Input: part model. Units: mm. Frame: model coordinates. Round coordinates to 2 decimals unless told otherwise and drop trailing zeros. Loops run counter-clockwise (first coordinate to the right, second up) from the corner with the lowest first, then second, coordinate; pieces in that order, holes last. Notation, with made-up numbers: (71, 9) - (98, 9) arc R10 ccw to (98, 13) - close; hole circle Ø10 at (-21.75, 8). An arc over 180 degrees is marked (long way). One line per question, with ' | ' between items. Start each with the question number.
Item 1: Material intervals for line 1 along Y through (x, z) = (0, -23.5); line 2 along Z through (x, y) = (-54.5, -18); line 3 along X through (y, z) = (11, -49.5), sorted ascending.
Item 2: First-contact query: pin 1 (6 mm diameter, centred on y = 30, z = -12.5, fed in from +X); pin 2 (3 mm diameter, centred on y = -22.5, z = -55, fed in from -X); pin 3 (1.5 mm diameter, centred on x = -29, y = -27, fed in from -Z). Flat tips, straight axial feed; report the tip coordinate or a pass-through.
Item 3: Section C-C, the plane z = 4. Return loops of the section in (x, y) (1 decimal), plus the area to 3 significant figures.
Item 4: Section A-A, the plane y = 0. Return loops of the section in (x, z), plus the area to 3 significant figures.
Item 5: Section B-B, the plane x = -11. Return loops of the section in (y, z), plus the area to 3 significant figures.
Item 6: Draft query along X for faces 1 (the face through (-16, -16, -76.2)), 2 (the face through (-139.695, 0.519, 6.261)), 3 (the face through (-126.2, 0.52, 6.44)). Return one class per face: pulls with the +X half, pulls with the -X half, needs draft (parallel to the pull), parting line crosses it, or undercut.
Item 7: Section D-D, the plane y = 17.5. Return loops of the section in (x, z).
```python
from build123d import *

# Parameters (mm, degrees)
BOSS_EXTRUDE1_DEPTH                                 = 12.7
CBORE_FOR_0_BINDING_HEAD_MACHINE_SCREW1_D           = 15.875
CBORE_FOR_0_BINDING_HEAD_MACHINE_SCREW1_CBORE_D     = 23.8252
CBORE_FOR_0_BINDING_HEAD_MACHINE_SCREW1_CBORE_DEPTH = 15.875
SKETCH9_R                                           = 20.6375
CUT_EXTRUDE2_DEPTH                                  = 146.358143907
SKETCH11_R                                          = 38.1
SKETCH11_R_2                                        = 20.6375
BOSS_EXTRUDE2_DEPTH                                 = 76.2


with BuildPart() as part:
    # Sketch1 → Boss-Extrude1 (new body)
    with BuildSketch(Plane.XY):
        with BuildLine():
            ThreePointArc((-117.122222222, 25.242722946), (-139.7, 0), (-117.122222222, -25.242722946))
            Line((-117.122222222, -25.242722946), (-4.233333333, -37.864084419))
            ThreePointArc((-4.233333333, -37.864084419), (38.1, 0), (-4.233333333, 37.864084419))
            Line((-4.233333333, 37.864084419), (-117.122222222, 25.242722946))
        make_face()
    extrude(amount=BOSS_EXTRUDE1_DEPTH)

    # CBORE for #0 Binding Head Machine Screw1 (through all)
    with Locations(Plane.XY.offset(12.7)):
        with Locations((-114.3, 0)):
            CounterBoreHole(CBORE_FOR_0_BINDING_HEAD_MACHINE_SCREW1_D / 2, CBORE_FOR_0_BINDING_HEAD_MACHINE_SCREW1_CBORE_D / 2, CBORE_FOR_0_BINDING_HEAD_MACHINE_SCREW1_CBORE_DEPTH)

    # Sketch9 → Cut-Extrude2 (cut, through all)
    with BuildSketch(Plane.XY.offset(12.7)):
        Circle(SKETCH9_R)
    extrude(amount=-CUT_EXTRUDE2_DEPTH, mode=Mode.SUBTRACT)

    # Sketch11 → Boss-Extrude2 (add)
    with BuildSketch(Plane(origin=(0, 0, 0), x_dir=(-1, 0, 0), z_dir=(0, 0, -1))):
        Circle(SKETCH11_R)
        with Locations(Location((0, 0, 0), (0, 0, 180))):
            Circle(SKETCH11_R_2, mode=Mode.SUBTRACT)
    extrude(amount=BOSS_EXTRUDE2_DEPTH)


solid = part.part
```
Return value:
1) line 1: -38.1 to -20.64, 20.64 to 38.1 | line 2: 0 to 12.7 | line 3: -36.48 to -17.46, 17.46 to 36.48
2) pin 1: x = 26.88 | pin 2: x = -31.79 | pin 3: z = 0
3) outline: (-117.1, -25.2) - (-4.2, -37.9) arc R38.1 ccw (long way) to (-4.2, 37.9) - (-117.1, 25.2) arc R25.4 ccw to start; hole circle Ø23.8 at (-114.3, 0); hole circle Ø41.3 at (0, 0) | area: 8,810 mm2
4) outline: (-139.7, 0) - (-126.21, 0) - (-126.21, 12.7) - (-139.7, 12.7) - close; (-102.39, 0) - (-38.1, 0) - (-38.1, -76.2) - (-20.64, -76.2) - (-20.64, 12.7) - (-102.39, 12.7) - close; (20.64, -76.2) - (38.1, -76.2) - (38.1, 12.7) - (20.64, 12.7) - close | area: 4,090 mm2
5) outline: (-37.11, 0) - (-36.48, 0) - (-36.48, -76.2) - (-17.46, -76.2) - (-17.46, 12.7) - (-37.11, 12.7) - close; (17.46, -76.2) - (36.48, -76.2) - (36.48, 0) - (37.11, 0) - (37.11, 12.7) - (17.46, 12.7) - close | area: 3,400 mm2
6) face 1: needs draft | face 2: pulls with the -X half | face 3: undercut
7) outline: (-132.71, 0) - (-33.84, 0) - (-33.84, -76.2) - (-10.94, -76.2) - (-10.94, 12.7) - (-132.71, 12.7) - close; (10.94, -76.2) - (33.84, -76.2) - (33.84, 12.7) - (10.94, 12.7) - close
